from build123d import *

# Parameters (mm, degrees)
SKETCH2_W                                       = 5
SKETCH2_H                                       = 227
BOSS_EXTRUDE1_DEPTH                             = 20
BOSS_EXTRUDE2_REACH                             = 277.987
CUT_EXTRUDE1_DEPTH                              = 44
F_3_0MM_DOWEL_HOLE1_D                           = 3
F_3_0MM_DOWEL_HOLE1_DEPTH                       = 3
F_3_0MM_DOWEL_HOLE1_TIP                         = 0.901290929
CSK_FOR_M3_FLAT_HEAD_MACHINE_SCREW1_D           = 3.4
CSK_FOR_M3_FLAT_HEAD_MACHINE_SCREW1_CSINK_D     = 6.3
CSK_FOR_M3_FLAT_HEAD_MACHINE_SCREW1_CSINK_ANGLE = 90
FILLET1_R                                       = 2.5


with BuildPart() as part:
    # Sketch2 → Boss-Extrude1 (new body)
    with BuildSketch(Plane.XY):
        Polygon((15, 12), (5, 12), (5, 232), (125, 232), (125, 12), (115, 12), (115, 0), (140, 0), (140, 237), (-10, 237), (-10, 0), (15, 0), align=None)
        with Locations((132.5, 118.5)):
            Rectangle(SKETCH2_W, SKETCH2_H, mode=Mode.SUBTRACT)
        with Locations((-2.5, 118.5)):
            Rectangle(SKETCH2_W, SKETCH2_H, mode=Mode.SUBTRACT)
    extrude(amount=BOSS_EXTRUDE1_DEPTH)

    # Boss-Extrude2: up to this face of the body (flat: up to its plane)
    boss_extrude2_end = Plane(part.part.faces().sort_by_distance((130, 118.5, 10))[0])
    # Sketch3 → Boss-Extrude2 (add, up to the picked face)
    with BuildSketch(Plane.ZY, mode=Mode.PRIVATE) as boss_extrude2_sk1:
        with BuildLine():
            Line((20, 0), (30, 0))
            Line((30, 0), (30, 2))
            ThreePointArc((30, 2), (22.928932188, 4.928932188), (20, 12))
            Line((20, 12), (20, 0))
        make_face()
    boss_extrude2_tool1 = split(extrude(boss_extrude2_sk1.sketch, amount=-BOSS_EXTRUDE2_REACH, mode=Mode.PRIVATE), bisect_by=boss_extrude2_end, keep=Keep.BOTH, mode=Mode.PRIVATE)
    # Sketch3 → Boss-Extrude2 (add, up to the picked face)
    with BuildSketch(Plane.ZY, mode=Mode.PRIVATE) as boss_extrude2_sk2:
        with BuildLine():
            Line((0, 0), (-10, 0))
            Line((-10, 0), (-10, 2))
            ThreePointArc((-10, 2), (-2.928932188, 4.928932188), (0, 12))
            Line((0, 12), (0, 0))
        make_face()
    boss_extrude2_tool2 = split(extrude(boss_extrude2_sk2.sketch, amount=-BOSS_EXTRUDE2_REACH, mode=Mode.PRIVATE), bisect_by=boss_extrude2_end, keep=Keep.BOTH, mode=Mode.PRIVATE)
    add(boss_extrude2_tool1.solids().sort_by(Axis((0, 2.673783, 23.568126), (1, 0, 0)))[0])
    add(boss_extrude2_tool2.solids().sort_by(Axis((0, 2.673783, -3.568126), (1, 0, 0)))[0])

    # Sketch4 → Cut-Extrude1 (cut)
    with BuildSketch(Plane.XY.offset(30)):
        with BuildLine():
            Line((15, 2), (15, 0))
            Line((15, 0), (115, 0))
            Line((115, 0), (115, 2))
            ThreePointArc((115, 2), (122.071067812, 4.928932188), (125, 12))
            Line((125, 12), (5, 12))
            ThreePointArc((5, 12), (7.928932188, 4.928932188), (15, 2))
        make_face()
    extrude(amount=-CUT_EXTRUDE1_DEPTH, mode=Mode.SUBTRACT)

    # Ø3.0mm Dowel Hole1
    with Locations(Plane.XZ):
        with Locations((7.5, 10), (122.5, 10)):
            Hole(F_3_0MM_DOWEL_HOLE1_D / 2, depth=F_3_0MM_DOWEL_HOLE1_DEPTH)
            with Locations((0, 0, -(F_3_0MM_DOWEL_HOLE1_DEPTH + F_3_0MM_DOWEL_HOLE1_TIP / 2))):  # 118° drill point
                Cone(0, F_3_0MM_DOWEL_HOLE1_D / 2, F_3_0MM_DOWEL_HOLE1_TIP, mode=Mode.SUBTRACT)

    # CSK for M3 Flat Head Machine Screw1 (through all)
    with Locations(Plane(origin=(0, 237, 0), x_dir=(1, 0, 0), z_dir=(0, 1, 0))):
        with Locations((40, -10), (90, -10), (65, -10)):
            CounterSinkHole(CSK_FOR_M3_FLAT_HEAD_MACHINE_SCREW1_D / 2, CSK_FOR_M3_FLAT_HEAD_MACHINE_SCREW1_CSINK_D / 2, counter_sink_angle=CSK_FOR_M3_FLAT_HEAD_MACHINE_SCREW1_CSINK_ANGLE)

    # Fillet1
    fillet1_edges = [part.edges().sort_by_distance(p)[0] for p in [
        (0, 232, 10),
        (-5, 232, 10),
        (-5, 5, 10),
        (130, 232, 10),
        (135, 232, 10),
        (135, 5, 10),
        (5, 232, 10),
        (125, 232, 10),
    ]]
    fillet(fillet1_edges, radius=FILLET1_R - 0.0001)  # a hair under: the kernel refuses the full size


solid = part.part
The listing builds one solid part. Answer for the finished solid, in the listing's coordinates (mm). A direction names the side the tool comes from. Give positions to 0.01 mm unless a question says otherwise; leave off trailing zeros. Order: outer loops, then holes, each group sorted by start corner. A loop starts at its lowest first (then second) coordinate and runs counter-clockwise, first axis right, second up. Notation, with made-up numbers: (-9.5, 41) - (31.5, 41) arc R15 ccw to (31.5, 45) - close; hole circle Ø3 at (72.25, 65). An arc over 180 degrees is marked (long way). One line per item, written item: value. Start each with the question number.
1) A cutting plane is placed at D-D on x = 29.5. Give the vertices of the cut face in (y, z).
2) A cutting plane is placed at C-C on x = 2.5. Give the vertices of the cut face in (y, z).
3) The mould has two halves that part along Y. Classify faces 1 (the face through (66, 237, 5)), 2 (the face through (130, 113, 10)), 3 (the face through (125, 0, 10)): released by +Y, released by -Y, zero draft, split by the parting line, or undercut.
4) A tool of negligible diameter and unlimited length cuts with its end or side. For faces 4 (the face through (5, 0, 10)), 5 (the face through (-5, 117, 10)), from which of +Z, -Z, +X, -X, +Y, -Y can it reach the whole face along a straight path? Write none if from no direction.
5) A cutting plane is placed at B-B on z = -3. Give the vertices of the cut face in (x, y).
6) Given pin 1 Ø2.5 at (x, z) = (40, 10) entering from +Y; pin 2 Ø1.5 at (x, z) = (103.5, 1.5) entering from -Y, each flat-ended and moving along its own axis, determine where each tip first touches the part or whether it passes through.
7) Find the intervals of material crossed by L1, parallel to X at y = 27.5, z = 11.5; L2, parallel to X at y = 0.7, z = 10; L3, parallel to Z at x = 40, y = 232.8, in increasing order.
8) A cutting plane is placed at A-A on y = 81. Give the vertices of the cut face in (x, z).
Answer sheet:
1. outline: (232, 0) - (237, 0) - (237, 20) - (232, 20) - close
2. outline: (0, -10) - (2, -10) arc R10 cw to (12, 0) - (237, 0) - (237, 20) - (12, 20) arc R10 cw to (2, 30) - (0, 30) - close
3. face 1: released by +Y
3. face 2: undercut
3. face 3: released by -Y
4. face 4: +Z, -Z, +X, -X, -Y
4. face 5: +Z, -Z
5. outline: (0, 0) - (15, 0) - (15, 2) arc R10 cw to (8, 4.86) - (0, 4.86) - close; (115, 0) - (130, 0) - (130, 4.86) - (122, 4.86) arc R10 cw to (115, 2) - close
6. pin 1: passes through
6. pin 2: stops at y = 232
7. L1: x = -10 to -5, 0 to 5, 125 to 130, 135 to 140
7. L2: x = -10 to 6, 9 to 15, 115 to 121, 124 to 140
7. L3: z = 0 to 8.3, 11.7 to 20
8. outline: (-10, 0) - (-5, 0) - (-5, 20) - (-10, 20) - close; (0, 0) - (5, 0) - (5, 20) - (0, 20) - close; (125, 0) - (130, 0) - (130, 20) - (125, 20) - close; (135, 0) - (140, 0) - (140, 20) - (135, 20) - close
